Here's how the part is built. I have some questions about the finished solid (model axes, mm). Round coordinates to 2 decimals unless told otherwise and drop trailing zeros. Write each loop counter-clockwise with the first axis right and the second up, starting at its lowest first coordinate (ties: lowest second). Pieces come first, ordered by that corner, then holes. Notation, with made-up numbers: (-34, -25) -> (-26, -25) arc R24 cw to (-26, 10) -> close; hole circle Ø11 at (27.25, -25.75). An arc over 180 degrees is marked (long way). Put each result on its own line as item: value. Start each with the question number.
1. Suppose I cut it at A-A (z = 0). Please give me the cut outline in (x, y).
2. I need wall thicknesses on probe 1 along X at (y, z) = (7, 0.5); probe 2 along Z at (x, y) = (-70, 5.5). Which ranges of each line are inside material? Lowest first, please. Write a range as from..to.
3. For pin 1 (3 mm diameter, centred on x = 125, z = 0, fed in from -Y); pin 2 (1 mm diameter, centred on x = 109, z = 1.5, fed in from -Y), each with a flat end and sliding along its axis, tell me the tip position at first contact or that it passes through.
4. Suppose I cut it at B-B (x = 70). Please give me the cut outline in (y, z).
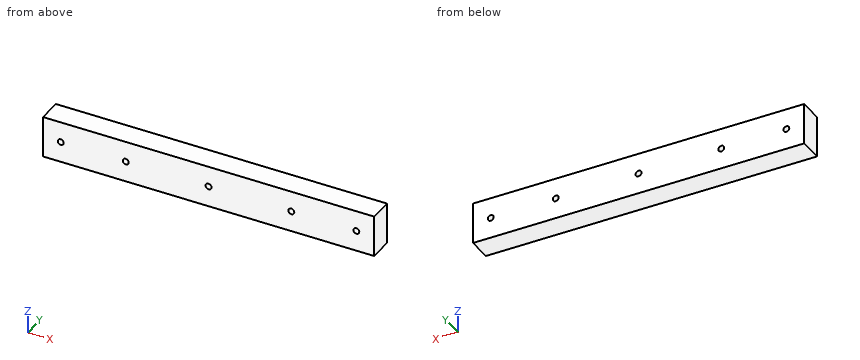
```python
from build123d import *

# Parameters (mm, degrees)
SKETCH1_W             = 280
SKETCH1_H             = 35
EXTRUDE1_DEPTH        = 20
M6_TAPPED_HOLE1_D     = 5
M6_TAPPED_HOLE1_DEPTH = 29
M6_TAPPED_HOLE1_TIP   = 1.502151548


with BuildPart() as part:
    # Sketch1 → Extrude1 (new body)
    with BuildSketch(Plane(origin=(0, 0, 0), x_dir=(1, 0, 0), z_dir=(0, 1, 0))):
        Rectangle(SKETCH1_W, SKETCH1_H)
    extrude(amount=EXTRUDE1_DEPTH)

    # M6 Tapped Hole1
    with Locations(Plane(origin=(0, 0, 0), x_dir=(-1, 0, 0), z_dir=(0, -1, 0))):
        with Locations((-125, 0), (-70, 0), (0, 0), (70, 0), (125, 0)):
            Hole(M6_TAPPED_HOLE1_D / 2, depth=M6_TAPPED_HOLE1_DEPTH)
            with Locations((0, 0, -(M6_TAPPED_HOLE1_DEPTH + M6_TAPPED_HOLE1_TIP / 2))):  # 118° drill point
                Cone(0, M6_TAPPED_HOLE1_D / 2, M6_TAPPED_HOLE1_TIP, mode=Mode.SUBTRACT)


solid = part.part
```
Verdict:
1. outline: (-140, 0) -> (-127.5, 0) -> (-127.5, 20) -> (-140, 20) -> close; (-122.5, 0) -> (-72.5, 0) -> (-72.5, 20) -> (-122.5, 20) -> close; (-67.5, 0) -> (-2.5, 0) -> (-2.5, 20) -> (-67.5, 20) -> close; (2.5, 0) -> (67.5, 0) -> (67.5, 20) -> (2.5, 20) -> close; (72.5, 0) -> (122.5, 0) -> (122.5, 20) -> (72.5, 20) -> close; (127.5, 0) -> (140, 0) -> (140, 20) -> (127.5, 20) -> close
2. probe 1: x = -140..-127.45, -122.55..-72.45, -67.55..-2.45, 2.45..67.55, 72.45..122.55, 127.45..140
2. probe 2: z = -17.5..-2.5, 2.5..17.5
3. pin 1: passes through
3. pin 2: stops at y = 0
4. outline: (0, -17.5) -> (20, -17.5) -> (20, -2.5) -> (0, -2.5) -> close; (0, 2.5) -> (20, 2.5) -> (20, 17.5) -> (0, 17.5) -> close
